Verification items for the finished model (mm, model axes). A direction names the side the tool comes from. Coordinates: 2 decimals unless noted, no trailing zeros. Loops run counter-clockwise (first coordinate to the right, second up) from the corner with the lowest first, then second, coordinate; pieces in that order, holes last.
Q1. Mould release check, pull along X, two halves, no side actions. Record for faces 1 (the face through (20, 20, 0)), 2 (the face through (6.11, 32.87, 1.97)), 3 (the face through (40, 20, 2)): +X half, -X half, draft (parallel to the pull), parting line (faces both ways), or undercut.
Q2. Access from +Z, -Z, +X, -X, +Y, -Y to the whole of each face (thin tool, end or side, straight path). Record for faces 4 (the face through (6.509, 9.656, 31.115)), 5 (the face through (0.57, 39.4, 2.03)).
Q3. Sectioned sample at D-D (z = 30). Enter the section's corners in (x, y).
Q4. Go/stop test with flat-tipped pins: P1, Ø10, axis at x = 22.5, z = 41.5, coming from the -Y side; P2, Ø17.5, axis at x = 18, y = 18, coming from the +Z side; P3, Ø6, axis at x = 4.5, z = 32.5, coming from the -Y side. Record where each tip stops, or that it passes through.
Q5. Sectioned sample at A-A (x = 20). Enter the section's corners in (y, z), then the cut area to 3 significant figures.
Q6. Sectioned sample at B-B (y = 35). Count the separate pieces of the cut face and the enclosed holes in it, then the cut area to 3 significant figures.
Q7. Material ranges on probe 1 along X at (y, z) = (5, 2); probe 2 along Z at (x, y) = (20.5, 21), recorded low to high.
```python
from build123d import *

# Parameters (mm, degrees)
CYLINDER004_R     = 17
CYLINDER004_DEPTH = 60
FILLET001_R       = 1
TORUS_R           = 1.5
CYLINDER_R        = 2.4
CYLINDER_DEPTH    = 10
CYLINDER001_R     = 2.4
CYLINDER001_DEPTH = 10
CYLINDER002_R     = 2.4
CYLINDER002_DEPTH = 10
CYLINDER003_R     = 2.4
CYLINDER003_DEPTH = 10
BOX_W             = 40
BOX_H             = 40
BOX_DEPTH         = 4
FILLET_R          = 2
FILLET002_R       = 1


with BuildPart() as cylinder004:
    # Cylinder004 → Cylinder004 (new body)
    with BuildSketch(Plane(origin=(20, 20, 0), x_dir=(1, 0, 0), z_dir=(0, 0, 1))):
        Circle(CYLINDER004_R)
    extrude(amount=CYLINDER004_DEPTH)


with BuildPart() as fillet001:
    # Fillet001 base: copy of Cylinder004
    add(cylinder004.part)

    # Fillet001
    fillet001_edges = [fillet001.edges().sort_by_distance(p)[0] for p in [
        (3, 20, 60),
    ]]
    fillet(fillet001_edges, radius=FILLET001_R)


with BuildPart() as cut001:
    # Torus → Torus (revolve)
    with BuildSketch(Plane(origin=(20, 20, 59), x_dir=(1, 0, 0), z_dir=(0, -1, 0))):
        with Locations((12, 0)):
            Circle(TORUS_R)
    revolve(axis=Axis((20, 20, 59), (0, 0, 1)))

    # Cut001: cut Fillet001
    add(fillet001.part, mode=Mode.SUBTRACT)


with BuildPart() as cylinder:
    # Cylinder → Cylinder (new body)
    with BuildSketch(Plane(origin=(5, 5, 0), x_dir=(1, 0, 0), z_dir=(0, 0, 1))):
        Circle(CYLINDER_R)
    extrude(amount=CYLINDER_DEPTH)


with BuildPart() as fusion:
    # Cylinder001 → Cylinder001 (new body)
    with BuildSketch(Plane(origin=(5, 35, 0), x_dir=(1, 0, 0), z_dir=(0, 0, 1))):
        Circle(CYLINDER001_R)
    extrude(amount=CYLINDER001_DEPTH)

    # Fusion: union Cylinder
    add(cylinder.part)


with BuildPart() as cylinder002:
    # Cylinder002 → Cylinder002 (new body)
    with BuildSketch(Plane(origin=(5, 5, 0), x_dir=(1, 0, 0), z_dir=(0, 0, 1))):
        Circle(CYLINDER002_R)
    extrude(amount=CYLINDER002_DEPTH)


with BuildPart() as fusion002:
    # Cylinder003 → Cylinder003 (new body)
    with BuildSketch(Plane(origin=(5, 35, 0), x_dir=(1, 0, 0), z_dir=(0, 0, 1))):
        Circle(CYLINDER003_R)
    extrude(amount=CYLINDER003_DEPTH)

    # Fusion001: union Cylinder002
    add(cylinder002.part)


with BuildPart() as fusion002_1:
    # Fusion001 placement: moved
    add(fusion002.part.moved(Location((30, 0, 0))))

    # Fusion002: union Fusion
    add(fusion.part)


with BuildPart() as cut:
    # Box → Box (new body)
    with BuildSketch(Plane.XY):
        with Locations((20, 20)):
            Rectangle(BOX_W, BOX_H)
    extrude(amount=BOX_DEPTH)

    # Fillet
    fillet_edges = [cut.edges().sort_by_distance(p)[0] for p in [
        (0, 0, 2),
        (0, 40, 2),
        (40, 0, 2),
        (40, 40, 2),
    ]]
    fillet(fillet_edges, radius=FILLET_R)

    # Cut: cut Fusion002
    add(fusion002_1.part, mode=Mode.SUBTRACT)


with BuildPart() as fusion003:
    # Fillet002 base: copy of Cylinder004
    add(cylinder004.part)

    # Fillet002
    fillet002_edges = [fusion003.edges().sort_by_distance(p)[0] for p in [
        (3, 20, 60),
    ]]
    fillet(fillet002_edges, radius=FILLET002_R)

    # Fusion003: union Cut001, Cut
    add(cut001.part)
    add(cut.part)


solid = fusion003.part
```
Geometry check:
1. face 1: draft
1. face 2: undercut
1. face 3: +X half
2. face 4: +Z
2. face 5: +Z, -Z, -X, +Y
3. outline: circle Ø34 at (20, 20)
4. P1: stops at y = 3
4. P2: stops at z = 60.44
4. P3: stops at y = 8.48
5. outline: (0, 0) - (40, 0) - (40, 4) - (37, 4) - (37, 59) arc R1 ccw to (36, 60) - (33.12, 60) arc R1.5 ccw to (30.88, 60) - (9.12, 60) arc R1.5 ccw to (6.88, 60) - (4, 60) arc R1 ccw to (3, 59) - (3, 4) - (0, 4) - close
5. area: 2,070 mm2
6. separate pieces: 3
6. enclosed holes: 0
6. area: 1,020 mm2
7. probe 1: x = 0 to 2.6, 7.4 to 32.6, 37.4 to 40
7. probe 2: z = 0 to 60
